```python
from build123d import *

# Parameters (mm, degrees)
SKETCH1_W           = 1368.425
SKETCH1_H           = 88.9
BOSS_EXTRUDE1_DEPTH = 38.1
CUT_EXTRUDE2_DEPTH  = 461.3021


with BuildPart() as part:
    # Sketch1 → Boss-Extrude1 (new body)
    with BuildSketch(Plane(origin=(0, 0, 0), x_dir=(1, 0, 0), z_dir=(0, 1, 0))):
        with Locations((0, 44.45)):
            Rectangle(SKETCH1_W, SKETCH1_H)
    extrude(amount=BOSS_EXTRUDE1_DEPTH)

    # Sketch3 → Cut-Extrude2 (cut, symmetric)
    with BuildSketch(Plane.ZY):
        with BuildLine():
            Line((-88.9, 0), (-70.192697288, 0))
            ThreePointArc((-70.192697288, 0), (-34.926054855, 2.738891811), (0, 8.343201677))
            Line((0, 8.343201677), (0, 38.1))
            Line((0, 38.1), (-88.9, 38.1))
            Line((-88.9, 38.1), (-88.9, 0))
        make_face()
    extrude(amount=CUT_EXTRUDE2_DEPTH, both=True, mode=Mode.SUBTRACT)


solid = part.part
```
The model under review builds one solid part; all positions refer to its coordinate system, in mm. A direction names the side the tool comes from. Coordinates: 2 decimals unless noted, no trailing zeros. Write each loop counter-clockwise with the first axis right and the second up, starting at its lowest first coordinate (ties: lowest second). Pieces come first, ordered by that corner, then holes. Notation, with made-up numbers: (-7, -11) -> (19, -11) arc R20 ccw to (19, 16) -> close; hole circle Ø5 at (71.25, 28). An arc over 180 degrees is marked (long way). One line per item, written item: value. Start each with the question number.
Q1. Clearance check with a flat-ended pin moving along its axis: P1, Ø10, axis at x = 342, z = -65.5, coming from the +Y side. State where the tip first meets the part, or that it passes through.
Q2. For faces 1 (the face through (-6.46, 2.68, -35.42)), 2 (the face through (571, 19, -88.9)), list the 3-axis set-ups (+Z, -Z, +X, -X, +Y, -Y) from which the entire face can be reached by the end or side of a thin tool; tool diameter is ignored.
Q3. To check wall thickness, follow probe 1 along X at (y, z) = (5, -40); probe 2 along Y at (x, z) = (-268.5, -65); probe 3 along Y at (x, z) = (-415.5, -4). State the ranges of each line that lie inside material, in increasing order.
Q4. Add section A-A, the plane y = 23.5. Give the boundary of the cut face in (x, z).
Q5. Add section B-B, the plane z = -57.5. Give the boundary of the cut face in (x, y), then the cut area to 3 significant figures.
Q6. The part is to be moulded in two halves that separate along X. For faces 3 (the face through (-461.302, 19, -45)), 4 (the face through (684.212, 19, -44)), 5 (the face through (-684.212, 19, -44)), 6 (the face through (-574, 19, -88.9)), say which applies: +X half, -X half, draft (parallel to the pull), parting line (faces both ways), or undercut.
Response:
1. P1: y = 0.46
2. face 1: -Z, +Y
2. face 2: -Z, +X, -X, +Y, -Y
3. probe 1: -684.21 to -461.3, 461.3 to 684.21
3. probe 2: 0 to 0.22
3. probe 3: 0 to 7.55
4. outline: (-684.21, -88.9) -> (-461.3, -88.9) -> (-461.3, 0) -> (-684.21, 0) -> close; (461.3, -88.9) -> (684.21, -88.9) -> (684.21, 0) -> (461.3, 0) -> close
5. outline: (-684.21, 0) -> (684.21, 0) -> (684.21, 38.1) -> (461.3, 38.1) -> (461.3, 0.65) -> (-461.3, 0.65) -> (-461.3, 38.1) -> (-684.21, 38.1) -> close
5. area: 17,600 mm²
6. face 3: undercut
6. face 4: +X half
6. face 5: -X half
6. face 6: draft
